from build123d import *

# Parameters (mm, degrees)
F0_W     = 1905
F0_H     = 1066.8
F1_DEPTH = 609.6
F3_DEPTH = 508


with BuildPart() as f1:
    # F0 (on Top) → F1 (new body)
    with BuildSketch(Plane.XY):
        Rectangle(F0_W, F0_H)
    extrude(amount=F1_DEPTH)

    # F2 (on face) → F3 (cut)
    with BuildSketch(Plane(origin=(0, 0, 0), x_dir=(1, 0, 0), z_dir=(0, 0, -1))):
        Polygon((952.5, -381), (952.5, 381), (800.1, 381), (800.1, 533.4), (-800.1, 533.4), (-800.1, 381), (-952.5, 381), (-952.5, -381), (-800.1, -381), (-800.1, -533.4), (800.1, -533.4), (800.1, -381), align=None)
    extrude(amount=-F3_DEPTH, mode=Mode.SUBTRACT)


solid = f1.part
Build history of the part. All positions in model axes, mm. A direction names the side the tool comes from. Coordinates: 2 decimals unless noted, no trailing zeros. Write each loop counter-clockwise with the first axis right and the second up, starting at its lowest first coordinate (ties: lowest second). Pieces come first, ordered by that corner, then holes.
(1) 3-axis set-ups, long thin cutter, end or side, ignore diameter. For faces 4 (the flat face through (800.1, -456, 250)), 5 (the flat face through (-877, 381, 250)), 6 (the flat face through (-4, -533.4, 552)): which of +Z, -Z, +X, -X, +Y, -Y reach the whole face in a straight line?
(2) Cut at C-C on y = -175.5. List the corners of the cut face in (x, z), and give its area (3 significant figures).
(3) Cut at B-B on x = 527. List the corners of the cut face in (y, z), and give its area (3 significant figures).
(4) Drill centre lines: line 1 (X direction, y = -457, z = 70); line 2 (Z direction, x = -369.5, y = -201). Where is each one in solid material? Low to high.
(5) Mould opens along Y. For faces 1 (the flat face through (-13, -7, 508)), 2 (the flat face through (-4, 533.4, 552)), 3 (the flat face through (952.5, -2, 529)) say: pulls with the +Y half, pulls with the -Y half, needs draft (parallel to the pull), parting line crosses it, or undercut.
(6) Cut at A-A on z = 423. List the corners of the cut face in (x, y), and give its area (3 significant figures).
(7) Pin check, flat tip, straight feed: pin 1 Ø2 at (x, y) = (-357.5, 82) entering from -Z. Stop position of the tip, or through.
Working result:
1. face 4: -Z, +Y, -Y
1. face 5: -Z, +X, -X
1. face 6: +Z, -Z, +X, -X, -Y
2. outline: (-952.5, 508) - (952.5, 508) - (952.5, 609.6) - (-952.5, 609.6) - close
2. area: 194,000 mm2
3. outline: (-533.4, 508) - (533.4, 508) - (533.4, 609.6) - (-533.4, 609.6) - close
3. area: 108,000 mm2
4. line 1: x = -952.5 to -800.1, 800.1 to 952.5
4. line 2: z = 508 to 609.6
5. face 1: undercut
5. face 2: pulls with the +Y half
5. face 3: needs draft
6. outline: (-952.5, -533.4) - (-800.1, -533.4) - (-800.1, -381) - (-952.5, -381) - close; (-952.5, 381) - (-800.1, 381) - (-800.1, 533.4) - (-952.5, 533.4) - close; (800.1, -533.4) - (952.5, -533.4) - (952.5, -381) - (800.1, -381) - close; (800.1, 381) - (952.5, 381) - (952.5, 533.4) - (800.1, 533.4) - close
6. area: 92,900 mm2
7. pin 1: stops at z = 508
